Verification items for the finished model (mm, model axes). Round coordinates to 2 decimals unless told otherwise and drop trailing zeros. Write each loop counter-clockwise with the first axis right and the second up, starting at its lowest first coordinate (ties: lowest second). Pieces come first, ordered by that corner, then holes. Notation, with made-up numbers: (24, 29) - (53, 29) arc R24 ccw to (53, 64) - close; hole circle Ø1 at (84, -25.75). An arc over 180 degrees is marked (long way). Answer as a JSON object with one key per item and string values.
```python
from build123d import *

# Parameters (mm, degrees)
ESBO_O1_R                = 1
ESBO_O1_R_2              = 1.4
ESBO_O1_R_3              = 1.5
RESSALTO_EXTRUS_O2_DEPTH = 4


with BuildPart() as part:
    # Esboço1 → Ressalto-extrusão2 (new body)
    with BuildSketch(Plane.XY):
        with BuildLine():
            Line((75.01453416, -40), (91.651513899, -40))
            ThreePointArc((91.651513899, -40), (0, -100), (-91.651513899, -40))
            Line((-91.651513899, -40), (-74.98546584, -40))
            Line((-74.98546584, -40), (-74.98546584, 40))
            Line((-74.98546584, 40), (-91.651513899, 40))
            ThreePointArc((-91.651513899, 40), (0, 100), (91.651513899, 40))
            Line((91.651513899, 40), (75.01453416, 40))
            Line((75.01453416, 40), (75.01453416, -40))
        make_face()
        with Locations((-57.5, 57.5)):
            Circle(ESBO_O1_R, mode=Mode.SUBTRACT)
        with Locations((57.5, 57.5)):
            Circle(ESBO_O1_R, mode=Mode.SUBTRACT)
        with Locations((57.5, -57.5)):
            Circle(ESBO_O1_R, mode=Mode.SUBTRACT)
        with Locations((-57.5, -57.5)):
            Circle(ESBO_O1_R, mode=Mode.SUBTRACT)
        with Locations((-46.9, 20)):
            Circle(ESBO_O1_R_2, mode=Mode.SUBTRACT)
        with Locations((46.92453416, 19.902879261)):
            Circle(ESBO_O1_R_2, mode=Mode.SUBTRACT)
        with Locations((-18.25, 95)):
            Circle(ESBO_O1_R_3, mode=Mode.SUBTRACT)
        with Locations((18.25, 95)):
            Circle(ESBO_O1_R_3, mode=Mode.SUBTRACT)
        with Locations((18.25, 58.5)):
            Circle(ESBO_O1_R_3, mode=Mode.SUBTRACT)
        with Locations((-18.25, 58.5)):
            Circle(ESBO_O1_R_3, mode=Mode.SUBTRACT)
        with Locations((-15, -95)):
            Circle(ESBO_O1_R_3, mode=Mode.SUBTRACT)
        with Locations((15, -95)):
            Circle(ESBO_O1_R_3, mode=Mode.SUBTRACT)
        with Locations((15, -72.5)):
            Circle(ESBO_O1_R_3, mode=Mode.SUBTRACT)
        with Locations((-15, -72.5)):
            Circle(ESBO_O1_R_3, mode=Mode.SUBTRACT)
        with Locations((-35.9, 20)):
            Circle(ESBO_O1_R_2, mode=Mode.SUBTRACT)
        with Locations((35.92453416, 20)):
            Circle(ESBO_O1_R_2, mode=Mode.SUBTRACT)
        Polygon((49.42453416, -5.097120739), (49.42453416, -12.097120739), (44.42453416, -12.097120739), (44.42453416, -5.097120739), (39.67453416, -5.097120739), (39.67453416, 0.902879261), (44.42453416, 0.902879261), (44.42453416, 7.902879261), (49.42453416, 7.902879261), (49.42453416, 0.902879261), (54.17453416, 0.902879261), (54.17453416, -5.097120739), align=None, mode=Mode.SUBTRACT)
        Polygon((-54.17453416, 0.902879261), (-54.17453416, -5.097120739), (-49.42453416, -5.097120739), (-49.42453416, -12.097120739), (-44.42453416, -12.097120739), (-44.42453416, -5.097120739), (-39.67453416, -5.097120739), (-39.67453416, 0.902879261), (-44.42453416, 0.902879261), (-44.42453416, 7.902879261), (-49.42453416, 7.902879261), (-49.42453416, 0.902879261), align=None, mode=Mode.SUBTRACT)
    extrude(amount=RESSALTO_EXTRUS_O2_DEPTH)


solid = part.part
```
1. Cross-section at A-A (y = 13). Record the boundary of the cut face in (x, z), plus the area to 3 significant figures.
Completed:
{"outline": "(-74.99, 0) - (75.01, 0) - (75.01, 4) - (-74.99, 4) - close", "area": "600 mm^2"}
2. Cross-section at B-B (z = 3.2). Count the separate pieces of the cut face and the enclosed holes in it, plus the area to 3 significant figures.
Completed:
{"separate pieces": "1", "enclosed holes": "18", "area": "27,400 mm^2"}
3. Material ranges on probe 1 along X at (y, z) = (-73, 1.6); probe 2 along Y at (x, z) = (15, 3); probe 3 along Y at (x, z) = (-18.25, 3), recorded low to high. Write a range as from..to.
Completed:
{"probe 1": "x = -68.34..-16.41, -13.59..13.59, 16.41..68.34", "probe 2": "y = -98.87..-96.5, -93.5..-74, -71..98.87", "probe 3": "y = -98.32..57, 60..93.5, 96.5..98.32"}
4. Go/stop test with flat-tipped pins: pin 1 (1.2 mm diameter, centred on x = 46.5, z = 1.5, fed in from -Y); pin 2 (2 mm diameter, centred on y = 2, z = 1, fed in from +X); pin 3 (2 mm diameter, centred on y = -1, z = 1, fed in from -X). Record where each tip stops, or that it passes through.
Completed:
{"pin 1": "stops at y = -88.84", "pin 2": "stops at x = 75.01", "pin 3": "stops at x = -74.99"}
5. Cross-section at C-C (y = -64). Record the boundary of the cut face in (x, z).
Completed:
{"outline": "(-76.84, 0) - (76.84, 0) - (76.84, 4) - (-76.84, 4) - close"}
